Could you check a few things on this model? Use its own coordinates, in mm. A direction names the side the tool comes from. Give positions to 0.01 mm unless a question says otherwise; leave off trailing zeros. Order: outer loops, then holes, each group sorted by start corner. A loop starts at its lowest first (then second) coordinate and runs counter-clockwise, first axis right, second up. Notation, with made-up numbers: M 87,46.5 L 109,46.5 A31 ccw 109,80.5 Z; hole C 40.25,73.25 d3. An arc over 180 degrees is marked long. Answer in a Markdown table with one row per item. Add a question column.
```python
from build123d import *

# Parameters (mm, degrees)
SKETCH1_W           = 60
SKETCH1_H           = 60
BOSS_EXTRUDE1_DEPTH = 50
CHAMFER1_SIZE       = 10
FILLET1_R           = 3
SHELL2_DEPTH        = 47
CUT_EXTRUDE1_REACH  = 100.489
SKETCH2_R           = 10
CUT_EXTRUDE2_DEPTH  = 5


# Read off the part's stored shape, not the designer's step: Shell2
with BuildPart() as part:
    # Sketch1 → Boss-Extrude1 (new body)
    with BuildSketch(Plane.XY):
        with Locations((30, 30)):
            Rectangle(SKETCH1_W, SKETCH1_H)
    extrude(amount=BOSS_EXTRUDE1_DEPTH)

    # Chamfer1
    chamfer1_edges = [part.edges().sort_by_distance(p)[0] for p in [
        (0, 60, 25),
        (60, 60, 25),
        (60, 0, 25),
        (0, 0, 25),
    ]]
    chamfer(chamfer1_edges, length=CHAMFER1_SIZE)

    # Fillet1
    fillet1_edges = [part.edges().sort_by_distance(p)[0] for p in [
        (0, 30, 50),
        (30, 60, 50),
        (30, 0, 50),
        (60, 30, 50),
        (55, 55, 50),
        (55, 5, 50),
        (5, 5, 50),
        (5, 55, 50),
    ]]
    fillet(fillet1_edges, radius=FILLET1_R)

    # Shell2 outline → Shell2 (cut)
    with BuildSketch(Plane.XY):
        Polygon((3, 48.757359313), (3, 11.242640687), (11.242640687, 3), (48.757359313, 3), (57, 11.242640687), (57, 48.757359313), (48.757359313, 57), (11.242640687, 57), align=None)
    extrude(amount=SHELL2_DEPTH, mode=Mode.SUBTRACT)

    # Sketch2 → Cut-Extrude1 (cut, up to next)
    with BuildSketch(Plane.XY.offset(50), mode=Mode.PRIVATE) as cut_extrude1_sk1:
        with Locations((30, 30)):
            Circle(SKETCH2_R)
    cut_extrude1_tool1 = extrude(cut_extrude1_sk1.sketch, amount=-CUT_EXTRUDE1_REACH, mode=Mode.PRIVATE) & part.part
    add(cut_extrude1_tool1.solids().sort_by_distance((30, 30, 50))[0], mode=Mode.SUBTRACT)

    # Sketch3 → Cut-Extrude2 (cut)
    with BuildSketch(Plane(origin=(0, 0, 0), x_dir=(-1, 0, 0), z_dir=(0, 0, -1))):
        Polygon((0, 10), (0, 50), (-10, 60), (-50, 60), (-60, 50), (-60, 10), (-50, 0), (-10, 0), align=None)
        Polygon((-1.5, 10.621320344), (-1.5, 49.378679656), (-10.621320344, 58.5), (-49.378679656, 58.5), (-58.5, 49.378679656), (-58.5, 10.621320344), (-49.378679656, 1.5), (-10.621320344, 1.5), align=None, mode=Mode.SUBTRACT)
    extrude(amount=-CUT_EXTRUDE2_DEPTH, mode=Mode.SUBTRACT)


solid = part.part
```
1. Suppose I cut it at A-A on x = 30. List the corners of the cut face in (y, z) for me.
2. Suppose I cut it at C-C on y = 27.5. List the corners of the cut face in (x, z) for me, plus the area to 3 significant figures.
3. Thinking about a two-plate mould opening in Y: for faces 1 (the flat face through (55, 5, 26)), 2 (the flat face through (53.88, 54, 2.46)), 3 (the flat face through (59, 30, 5)), 4 (the flat face through (30, 57, 23)), which applies, pulls with the +Y half, pulls with the -Y half, needs draft (parallel to the pull), parting line crosses it, or undercut?
4. Suppose I cut it at B-B on z = 9. List the corners of the cut face in (x, y) for me.
5. For faces 5 (the flat face through (6, 53.88, 2.46)), 6 (the flat face through (6.12, 6, 2.46)), 7 (the flat face through (1.5, 30, 2)), 8 (the flat face through (52.94, 52.82, 23.17)), which set-ups out of +Z, -Z, +X, -X, +Y, -Y let a thin tool reach every point of the face, with its end or its side?
6. Suppose I cut it at D-D on y = 18.5. List the corners of the cut face in (x, z) for me.
7. Will these pins go through, and if not, where does the flat tip stop? P1, Ø5.5, axis at y = 35, z = 3.5, coming from the +X side; P2, Ø12, axis at x = 24, y = 25.5, coming from the -Z side; P3, Ø1.5, axis at y = 36, z = 1.5, coming from the -X side; P4, Ø1.5, axis at x = 38.5, z = 2.5, coming from the +Y side.
8. If I drill on line 1 along X through (y, z) = (24.5, 36.5); line 2 along Y through (x, z) = (13.5, 3.5), over which ranges is the centre line in solid material (lowest first)? Write a range as [from, to].
Findings below:
| question | item | result |
|---|---|---|
| 1 | outline | M 0,5 L 1.5,5 L 1.5,0 L 3,0 L 3,47 L 20,47 L 20,50 L 3,50 A3 ccw 0,47 Z; M 40,47 L 57,47 L 57,0 L 58.5,0 L 58.5,5 L 60,5 L 60,47 A3 ccw 57,50 L 40,50 Z |
| 2 | outline | M 0,5 L 1.5,5 L 1.5,0 L 3,0 L 3,47 L 20.32,47 L 20.32,50 L 3,50 A3 ccw 0,47 Z; M 39.68,47 L 57,47 L 57,0 L 58.5,0 L 58.5,5 L 60,5 L 60,47 A3 ccw 57,50 L 39.68,50 Z |
| 2 | area | 385 mm2 |
| 3 | face 1 | pulls with the -Y half |
| 3 | face 2 | pulls with the +Y half |
| 3 | face 3 | needs draft |
| 3 | face 4 | undercut |
| 4 | outline | M 0,10 L 10,0 L 50,0 L 60,10 L 60,50 L 50,60 L 10,60 L 0,50 Z; hole M 3,11.24 L 11.24,3 L 48.76,3 L 57,11.24 L 57,48.76 L 48.76,57 L 11.24,57 L 3,48.76 Z |
| 5 | face 5 | -Z, -X, +Y |
| 5 | face 6 | -Z, -X, -Y |
| 5 | face 7 | -Z, -X, +Y, -Y |
| 5 | face 8 | -Z |
| 6 | outline | M 0,5 L 1.5,5 L 1.5,0 L 3,0 L 3,47 L 57,47 L 57,0 L 58.5,0 L 58.5,5 L 60,5 L 60,47 A3 ccw 57,50 L 3,50 A3 ccw 0,47 Z |
| 7 | P1 | x = 60 |
| 7 | P2 | z = 47 |
| 7 | P3 | x = 1.5 |
| 7 | P4 | y = 58.5 |
| 8 | line 1 | [0, 3], [57, 60] |
| 8 | line 2 | [1.5, 3], [57, 58.5] |
